```python
from build123d import *

# Parameters (mm, degrees)
BOSS_EXTRUDE2_DEPTH = 3
BOSS_EXTRUDE3_DEPTH = 25
SKETCH3_W           = 3
SKETCH3_H           = 20
BOSS_EXTRUDE4_DEPTH = 25
SKETCH4_R           = 7.5
CUT_EXTRUDE1_DEPTH  = 6
CUT_EXTRUDE2_DEPTH  = 6
SKETCH6_R           = 5
CUT_EXTRUDE3_DEPTH  = 6
SKETCH7_R           = 2
CUT_EXTRUDE4_DEPTH  = 153


with BuildPart() as part:
    # Sketch2 → Boss-Extrude2 (new body)
    # profile 1 of 2: a face of its own
    with BuildSketch(Plane.XY):
        Polygon((-11.333647929, 47), (-11.333647929, 97), (76.666352071, 97), (76.666352071, 47), (67.850003036, -3), (-2.517298894, -3), align=None)
        Polygon((0, 0), (-8.333647929, 47.262465991), (-8.333647929, 94), (73.666352071, 94), (73.666352071, 47.262465991), (65.332704142, 0), align=None, mode=Mode.SUBTRACT)
    # profile 2 of 2: a face of its own
    with BuildSketch(Plane.XY):
        Polygon((-8.333647929, 47.262465991), (-8.333647929, 94), (73.666352071, 94), (73.666352071, 47.262465991), (65.332704142, 0), (0, 0), align=None)
    extrude(amount=BOSS_EXTRUDE2_DEPTH)

    # Sketch2<4> → Boss-Extrude3 (add)
    with BuildSketch(Plane.XY):
        Polygon((-11.333647929, 97), (76.666352071, 97), (76.666352071, 47), (67.850003036, -3), (-2.517298894, -3), (-11.333647929, 47), align=None)
        Polygon((-8.333647929, 94), (73.666352071, 94), (73.666352071, 47.262465991), (65.332704142, 0), (0, 0), (-8.333647929, 47.262465991), align=None, mode=Mode.SUBTRACT)
    extrude(amount=BOSS_EXTRUDE3_DEPTH)

    # Sketch3 → Boss-Extrude4 (add)
    with BuildSketch(Plane(origin=(0, 0, 0), x_dir=(-1, 0, 0), z_dir=(0, 0, -1))):
        with Locations((9.833647929, 107)):
            Rectangle(SKETCH3_W, SKETCH3_H)
        with Locations((-11.416352071, 107)):
            Rectangle(SKETCH3_W, SKETCH3_H)
        with Locations((-32.666352071, 107)):
            Rectangle(SKETCH3_W, SKETCH3_H)
        with Locations((-53.916352071, 107)):
            Rectangle(SKETCH3_W, SKETCH3_H)
        with Locations((-75.166352071, 107)):
            Rectangle(SKETCH3_W, SKETCH3_H)
    extrude(amount=-BOSS_EXTRUDE4_DEPTH)

    # Sketch4 → Cut-Extrude1 (cut)
    with BuildSketch(Plane(origin=(66.317105319, -11.69349495, 0), x_dir=(0, 0, -1), z_dir=(0.9848077530122088, -0.17364817766692645, 0))):
        with Locations(Location((-12.5, 29.630807288, 0), (0, 0, 90))):
            Circle(SKETCH4_R)
    extrude(amount=-CUT_EXTRUDE1_DEPTH, mode=Mode.SUBTRACT)

    # Sketch5 → Cut-Extrude2 (cut)
    with BuildSketch(Plane.XZ.offset(3)):
        with BuildLine():
            Line((47.666352071, 7.5), (17.666352071, 7.5))
            ThreePointArc((17.666352071, 7.5), (12.666352071, 12.5), (17.666352071, 17.5))
            Line((17.666352071, 17.5), (47.666352071, 17.5))
            ThreePointArc((47.666352071, 17.5), (52.666352071, 12.5), (47.666352071, 7.5))
        make_face()
    extrude(amount=-CUT_EXTRUDE2_DEPTH, mode=Mode.SUBTRACT)

    # Sketch6 → Cut-Extrude3 (cut)
    with BuildSketch(Plane(origin=(0, 97, 0), x_dir=(1, 0, 0), z_dir=(0, 1, 0))):
        with Locations(Location((0.791352071, -12.5, 0), (0, 0, 270))):
            Circle(SKETCH6_R)
        with Locations(Location((22.041352071, -12.5, 0), (0, 0, 270))):
            Circle(SKETCH6_R)
        with Locations(Location((43.291352071, -12.5, 0), (0, 0, 270))):
            Circle(SKETCH6_R)
        with Locations(Location((64.541352071, -12.5, 0), (0, 0, 270))):
            Circle(SKETCH6_R)
    extrude(amount=-CUT_EXTRUDE3_DEPTH, mode=Mode.SUBTRACT)

    # Sketch7 → Cut-Extrude4 (cut)
    with BuildSketch(Plane.ZY.offset(11.333647929)):
        with Locations((12.5, 107)):
            Circle(SKETCH7_R)
    extrude(amount=-CUT_EXTRUDE4_DEPTH, mode=Mode.SUBTRACT)


solid = part.part
```
The model under review builds one solid part; all positions refer to its coordinate system, in mm. A direction names the side the tool comes from. Coordinates: 2 decimals unless noted, no trailing zeros. Write each loop counter-clockwise with the first axis right and the second up, starting at its lowest first coordinate (ties: lowest second). Pieces come first, ordered by that corner, then holes. Notation, with made-up numbers: (53.5, -27.5) - (78.5, -27.5) arc R28 ccw to (78.5, 0.5) - close; hole circle Ø10 at (78.5, 65). An arc over 180 degrees is marked (long way). Answer in a Markdown table with one row per item. Add a question column.
Q1. To check wall thickness, follow line 1 along X through (y, z) = (108, 17); line 2 along X through (y, z) = (59.5, 12.25); line 3 along Y through (x, z) = (53.25, 12.5). State the ranges of each line that lie inside material, in increasing order. Write a range as from..to.
Q2. Draft analysis for pull direction Y (two halves, no side actions). For faces 5 (the face through (-6.864, 21.65, 12.325)), 6 (the face through (69.72, 16.14, 5.18)), 7 (the face through (76.666, 82, 12)), state which applies: +Y half, -Y half, draft (parallel to the pull), parting line (faces both ways), or undercut.
Q3. Consider section A-A on y = 81. Give the boundary of the cut face in (x, z).
Q4. Clearance check with flat-ended pins moving along their axes: pin 1 (1.5 mm diameter, centred on x = 42, z = 6, fed in from +Y); pin 2 (2 mm diameter, centred on x = 58, y = 37.5, fed in from +Z). State where each tip first meets the part, or that it passes through.
Q5. Consider section D-D on z = 12.5. Give the number of separate pieces and of enclosed holes in the cut face, then the cut area to 3 significant figures.
Q6. For faces 1 (the face through (52.665, -1.521, 12.61)), 2 (the face through (2.29, 95.52, 17.27)), 3 (the face through (52.416, 104.6, 12.3)), 4 (the face through (38.855, 95.521, 14.807)), list the 3-axis set-ups (+Z, -Z, +X, -X, +Y, -Y) from which the entire face can be reached by the end or side of a thin tool; tool diameter is ignored.
Q7. Consider section B-B on y = 95.5. Give the boundary of the cut face in (x, z).
Answers below:
| question | item | result |
|---|---|---|
| 1 | line 1 | -11.33..-8.33, 9.92..12.92, 31.17..34.17, 52.42..55.42, 73.67..76.67 |
| 1 | line 2 | -11.33..-8.33, 73.67..76.67 |
| 1 | line 3 | -3..0, 94..105, 109..117 |
| 2 | face 5 | -Y half |
| 2 | face 6 | undercut |
| 2 | face 7 | draft |
| 3 | outline | (-11.33, 0) - (76.67, 0) - (76.67, 25) - (73.67, 25) - (73.67, 3) - (-8.33, 3) - (-8.33, 25) - (-11.33, 25) - close |
| 4 | pin 1 | y = 97 |
| 4 | pin 2 | z = 3 |
| 5 | separate pieces | 11 |
| 5 | enclosed holes | 0 |
| 5 | area | 1,000 mm² |
| 6 | face 1 | -Y |
| 6 | face 2 | +Y |
| 6 | face 3 | +Z, -Z, +Y |
| 6 | face 4 | +Y, -Y |
| 7 | outline | (-11.33, 0) - (76.67, 0) - (76.67, 25) - (-11.33, 25) - close; hole circle Ø10 at (0.79, 12.5); hole circle Ø10 at (22.04, 12.5); hole circle Ø10 at (43.29, 12.5); hole circle Ø10 at (64.54, 12.5) |
